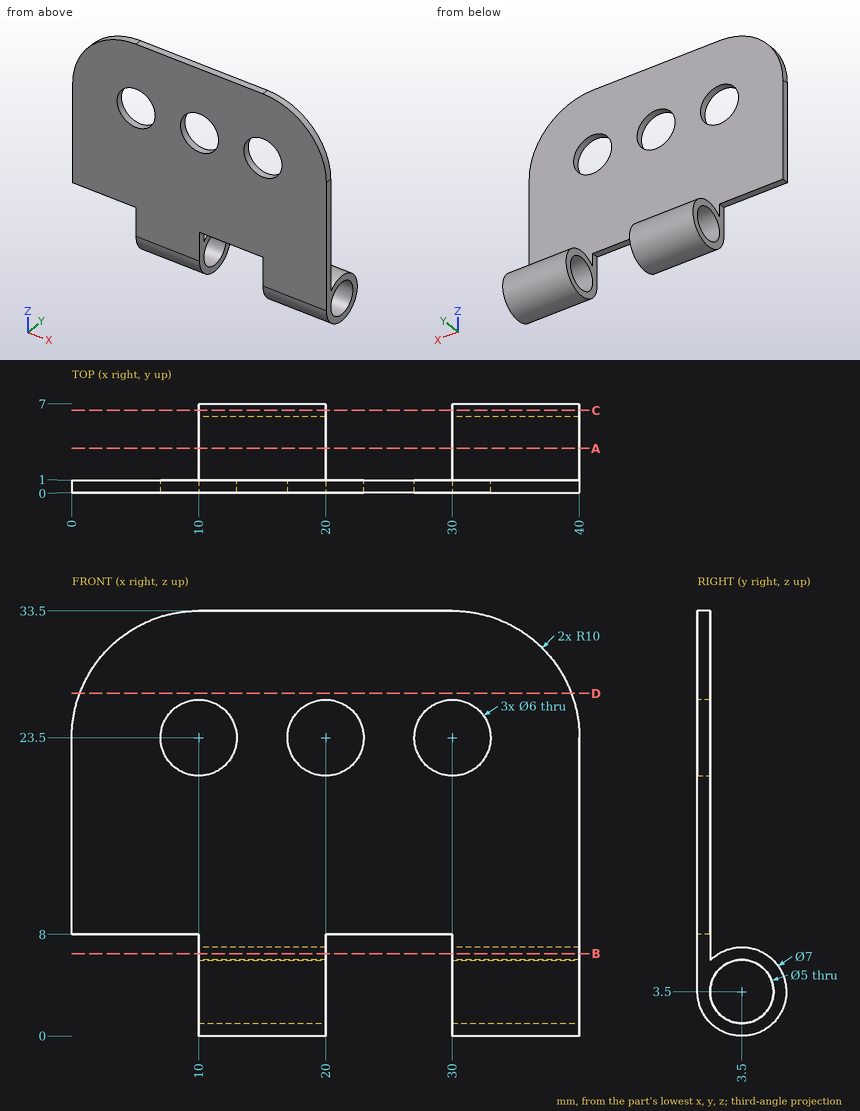
For this review, use the dimensioned drawing (mm, ordinates from the lowest corner) and the shaded views. Round coordinates to 2 decimals unless told otherwise and drop trailing zeros. Order: outer loops, then holes, each group sorted by start corner. A loop starts at its lowest first (then second) coordinate and runs counter-clockwise, first axis right, second up. Notation, with made-up numbers: M 49.5,19 L 78.5,19 A22 ccw 78.5,56 Z; hole C -28.75,37 d5. An arc over 180 degrees is marked long. Use a Markdown table: item, result.
1) Consider section A-A (y = 3.5). Write out the cut boundary in (x, z), then the cut area to 3 significant figures.
Report:
| item | result |
|---|---|
| outline | M 10,0 L 20,0 L 20,1 L 10,1 Z; M 10,6 L 20,6 L 20,7 L 10,7 Z; M 30,0 L 40,0 L 40,1 L 30,1 Z; M 30,6 L 40,6 L 40,7 L 30,7 Z |
| area | 40.0 mm^2 |
2) Wall thickness on line 1 along Y through (x, z) = (30.5, 20.5); line 2 along X through (y, z) = (6.75, 4); line 3 along Z through (x, y) = (17, 3.75): over which ranges is each line inside the solid? List them lowest first. Write a range as [from, to].
Report:
| item | result |
|---|---|
| line 1 | [0, 1] |
| line 2 | [10, 20], [30, 40] |
| line 3 | [0.01, 1.01], [5.99, 6.99] |
3) Consider section B-B (z = 6.5). Write out the cut boundary in (x, y), then the cut area to 3 significant figures.
Report:
| item | result |
|---|---|
| outline | M 10,0 L 20,0 L 20,1 L 10,1 Z; M 10,1.7 L 20,1.7 L 20,5.3 L 10,5.3 Z; M 30,0 L 40,0 L 40,1 L 30,1 Z; M 30,1.7 L 40,1.7 L 40,5.3 L 30,5.3 Z |
| area | 92.1 mm^2 |
4) Consider section C-C (y = 6.5). Write out the cut boundary in (x, z), then the cut area to 3 significant figures.
Report:
| item | result |
|---|---|
| outline | M 10,1.7 L 20,1.7 L 20,5.3 L 10,5.3 Z; M 30,1.7 L 40,1.7 L 40,5.3 L 30,5.3 Z |
| area | 72.1 mm^2 |
5) Insertion check: pin 1 (5 mm diameter, centred on x = 30, z = 23.5, fed in from -Y); pin 2 (6 mm diameter, centred on x = 24, z = 17.5, fed in from +Y); pin 3 (3.5 mm diameter, centred on y = 5, z = 2.5, fed in from -X). Each pin has a flat end and moves straight along its axis. Give the tip position at first contact, or say it passes through.
Report:
| item | result |
|---|---|
| pin 1 | through |
| pin 2 | y = 1 |
| pin 3 | x = 10 |
6) Consider section D-D (z = 27). Write out the cut boundary in (x, y), then the cut area to 3 significant figures.
Report:
| item | result |
|---|---|
| outline | M 0.63,0 L 39.37,0 L 39.37,1 L 0.63,1 Z |
| area | 38.7 mm^2 |
